Work out the finished part from the listing and answer in its coordinate system (mm). A direction names the side the tool comes from. Round coordinates to 2 decimals unless told otherwise and drop trailing zeros. Write each loop counter-clockwise with the first axis right and the second up, starting at its lowest first coordinate (ties: lowest second). Pieces come first, ordered by that corner, then holes. Notation, with made-up numbers: (18, -3.5) -> (50, -3.5) arc R22 cw to (50, 29.5) -> close; hole circle Ø7 at (5, 36). An arc over 180 degrees is marked (long way). Answer as a JSON object with one key per item and string values. Group by question number.
from build123d import *

# Parameters (mm, degrees)
EXTRUDE_1_DEPTH     = 5
CUT_EXTRUDE_1_REACH = 54.767
SKETCH_2_R          = 7.75
SKETCH_3_R          = 9.5
CUT_EXTRUDE_2_DEPTH = 2
CUT_EXTRUDE_START   = -2
SKETCH_4_R          = 9.5
CUT_EXTRUDE_3_DEPTH = 2
FILLET_1_R          = 1


with BuildPart() as part:
    # 草图1 → 凸台-拉伸1 (new body)
    with BuildSketch(Plane(origin=(0, 0, 0), x_dir=(1, 0, 0), z_dir=(0, 1, 0))):
        with BuildLine():
            Line((-38.520408163, 12.5), (38.520408163, 12.5))
            ThreePointArc((38.520408163, 12.5), (51.020408163, 0), (38.520408163, -12.5))
            Line((38.520408163, -12.5), (-38.520408163, -12.5))
            ThreePointArc((-38.520408163, -12.5), (-51.020408163, 0), (-38.520408163, 12.5))
        make_face()
    extrude(amount=EXTRUDE_1_DEPTH)

    # 草图2 → 切除-拉伸1 (cut, up to next)
    with BuildSketch(Plane(origin=(0, 5, 0), x_dir=(1, 0, 0), z_dir=(0, 1, 0)), mode=Mode.PRIVATE) as cut_extrude_1_sk1:
        with Locations(Location((38.520408163, 0, 0), (0, 0, 270))):
            Circle(SKETCH_2_R)
    cut_extrude_1_tool1 = extrude(cut_extrude_1_sk1.sketch, amount=-CUT_EXTRUDE_1_REACH, mode=Mode.PRIVATE) & part.part
    add(cut_extrude_1_tool1.solids().sort_by_distance((38.520408, 5, 0))[0], mode=Mode.SUBTRACT)

    # 草图3 → 切除-拉伸2 (cut)
    with BuildSketch(Plane(origin=(0, 5, 0), x_dir=(1, 0, 0), z_dir=(0, 1, 0))):
        with Locations(Location((38.520408163, 0, 0), (0, 0, 270))):
            Circle(SKETCH_3_R)
    extrude(amount=-CUT_EXTRUDE_2_DEPTH, mode=Mode.SUBTRACT)

    # 草图4 → 切除-拉伸3 (cut)
    with BuildSketch(Plane.XZ.offset(CUT_EXTRUDE_START)):
        with Locations(Location((38.520408163, 0, 0), (0, 0, 90))):
            Circle(SKETCH_4_R)
    extrude(amount=CUT_EXTRUDE_3_DEPTH, mode=Mode.SUBTRACT)

    # 圆角1
    fillet_1_edges = [part.edges().sort_by_distance(p)[0] for p in [
        (38.520408163, 3, -9.5),
        (38.520408163, 2, -9.5),
    ]]
    fillet(fillet_1_edges, radius=FILLET_1_R)


solid = part.part
1) Straight lines are drawn through the part: L1, parallel to X at y = 0.25, z = 0; L2, parallel to X at y = 2.8, z = 0; L3, parallel to Z at x = 43.5, y = 1.1. For each, find the intervals that lie inside material, in ascending order.
2) A tool of negligible diameter and unlimited length cuts with its end or side. For faces 4 (the face through (29.1, 0.51, -1.24)), 5 (the face through (46.53, 4.51, 5.11)), 6 (the face through (46.204, 2.507, -1.009)), from which of +Z, -Z, +X, -X, +Y, -Y can it reach the whole face along a straight path? Write none if from no direction.
3) A cutting plane is placed at A-A on z = 0. Determine the outline of the cut face in (x, y), plus the area to 3 significant figures.
4) This flat-tipped pin is pushed along its axis until it touches: P1, Ø1.5, axis at y = 1.5, z = -2.5, coming from the +X side. Where does it stop, or does it pass through?
5) For a pull along Z with two mould halves and no side action, classify faces 1 (the face through (1, 2, 12.5)), 2 (the face through (37, 2, 8)), 3 (the face through (-11, 5, 0)) as released by +Z, released by -Z, zero draft, split by the parting line, or undercut.
Established:
{
 "1": {"L1": "x = -51.02 to 29.02, 48.02 to 51.02", "L2": "x = -51.02 to 30.77, 46.27 to 51.02", "L3": "z = -11.47 to -8.08, 8.08 to 11.47"},
 "2": {"face 4": "-Y", "face 5": "+Y", "face 6": "+Y, -Y"},
 "3": {"outline": "(-51.02, 0) -> (29.02, 0) -> (29.02, 1) arc R1 cw to (30.02, 2) -> (30.77, 2) -> (30.77, 3) -> (30.02, 3) arc R1 cw to (29.02, 4) -> (29.02, 5) -> (-51.02, 5) -> close; (46.27, 2) -> (47.02, 2) arc R1 cw to (48.02, 1) -> (48.02, 0) -> (51.02, 0) -> (51.02, 5) -> (48.02, 5) -> (48.02, 4) arc R1 cw to (47.02, 3) -> (46.27, 3) -> close", "area": "420 mm²"},
 "4": {"P1": "stops at x = 50.9"},
 "5": {"face 1": "released by +Z", "face 2": "undercut", "face 3": "zero draft"}
}
